Model file for the job. Use its own axes, mm. A direction names the side the tool comes from. Give positions to 0.01 mm unless a question says otherwise; leave off trailing zeros. Loops run counter-clockwise (first coordinate to the right, second up) from the corner with the lowest first, then second, coordinate; pieces in that order, holes last. Notation, with made-up numbers: M 45,9 L 86,9 A27 ccw 86,34 Z; hole C 29,73 d6. An arc over 180 degrees is marked long. Answer in a Markdown table with one row per item.
Autodesk Inventor part; units mm, degrees
ref_plane "Work Plane1" through (-4, 29, 0) normal (0, 1, 0) x (1, 0, 0)
ref_plane "Work Plane2" through (22.5, -4, 10) normal (1, 0, 0) x (0, 0, -1)
ref_plane "YZ Plane" through (0, 0, 0) normal (1, 0, 0) x (0, 1, 0)
sketch "Sketch1" plane through (0, 0, 0) normal (0, 0, 1) x (1, 0, 0)
  line L0 (0, 0) -> (45, 0)
  line L1 (45, 0) -> (45, 58)
  line L2 (45, 58) -> (0, 58)
  line L3 (0, 58) -> (0, 0)
  circle A0 centre (22.5, 53) radius 2.75
  circle A1 centre (22.5, 5) radius 2.75
  line L4 (19.75, 58) -> (19.75, 53)
  line L5 (25.25, 58) -> (25.25, 53)
  line L6 (0, 42) -> (45, 42)
  line L7 (45, 42) -> (45, 16)
  line L8 (45, 16) -> (0, 16)
  line L9 (0, 16) -> (0, 42)
  circle A2 centre (22.5, 53) radius 6
  circle A3 centre (22.5, 5) radius 6
  line L10 (16.5, 5) -> (16.5, -1)
  line L11 (28.5, 5) -> (28.5, -1)
  line L12 (16.5, 53) -> (16.5, 59)
  line L13 (28.5, 53) -> (28.5, 59)
  line L14 (-1, 59) -> (46, 59)
  line L15 (46, 59) -> (46, -1)
  line L16 (46, -1) -> (-1, -1)
  line L17 (-1, -1) -> (-1, 59)
  line L18 (49, 62) -> (-4, 62)
  line L19 (-4, 62) -> (-4, -4)
  line L20 (-4, -4) -> (49, -4)
  line L21 (49, -4) -> (49, 62)
  line L22 (28.5, 59) -> (16.5, 59)
  line L23 (28.5, -1) -> (16.5, -1)
  point P0 (22.5, 58)
  dimension "d0" = 45
  dimension "d1" = 58
  dimension "d2" = 5.5
  dimension "d3" = 5.5
  dimension "d4" = 5
  dimension "d5" = 5
  dimension "d6" = 26
  dimension "d7" = 16
  dimension "d8" = 12
  dimension "d9" = 12
  dimension "d10" = 1
  dimension "d11" = 3
extrude "Extrusion1" add sketch "Sketch1" along normal blind 10 contours L21 L20 L19 L18
sketch "Sketch2" plane through (0, 0, 10) normal (0, 0, 1) x (1, 0, 0)
  line L0 (-1, 59) -> (46, 59)
  line L1 (46, 59) -> (46, -1)
  line L2 (-1, 59) -> (46, 59)
  line L3 (46, 59) -> (46, 43)
  line L4 (46, 43) -> (-1, 43)
  line L5 (-1, 43) -> (-1, 59)
  line L6 (-1, -1) -> (-1, 59)
  line L7 (46, -1) -> (-1, -1)
  line L8 (-1, -1) -> (-1, 15)
  line L9 (-1, 15) -> (46, 15)
  line L10 (46, 15) -> (46, -1)
  point P0 (0, 0)
  dimension "d14" = 16
  dimension "d15" = 16
extrude "Extrusion2" add sketch "Sketch2" against normal blind 3 contours L0 L1 L4 L5 | L9 L1 L7 L6
sketch "Sketch3" plane through (0, 0, 0) normal (0, 0, -1) x (-1, 0, 0)
  arc A0 (-28.5, 53) -> (-16.5, 53) centre (-22.5, 53) ccw
  line L0 (-46, 59) -> (1, 59)
  line L1 (-28.5, 59) -> (-28.5, 53)
  line L2 (-16.5, 59) -> (-16.5, 53)
  line L3 (-16.5, 59) -> (-28.5, 59)
  point P0 (0, 0)
  dimension "d18" = 12
extrude "Extrusion3" add sketch "Sketch3" against normal up to surface (7 mm away)
ref_plane "Work Plane1" through (-4, 29, 0) normal (0, 1, 0) x (1, 0, 0)
mirror "Mirror1" about plane through (-4, 29, 0) normal (0, 1, 0) of "Extrusion3"
thicken "Thicken1" operation add thickness 13 both sides no extend neighbours yes toward (0, 0, -1) faces at (48, 39, 0)
sketch "Sketch4" plane through (-4, 62, 10) normal (0, 1, 0) x (1, 0, 0)
  line L0 (3, 3) -> (3, 0)
  line L1 (3, 0) -> (3, 3)
  line L2 (3, 23) -> (3, 3)
  line L3 (3, 23) -> (3, 3)
  line L4 (50, 0) -> (50, 3)
  line L5 (50, 23) -> (50, 3)
  line L6 (50, 23) -> (50, 3)
  line L7 (50, 3) -> (50, 0)
  line L8 (20.5, 3) -> (32.5, 3)
  line L9 (50, 3) -> (32.5, 3)
  line L10 (50, 3) -> (3, 3)
  line L11 (20.5, 3) -> (3, 3)
  line L12 (32.5, 23) -> (32.5, 3)
  line L13 (32.5, 23) -> (32.5, 3)
  line L14 (20.5, 23) -> (20.5, 3)
  line L15 (20.5, 3) -> (20.5, 23)
  line L16 (53, 23) -> (0, 23)
  line L17 (42, 23) -> (42, 7) construction
  line L18 (38, 23) -> (38, 7)
  line L19 (46, 7) -> (46, 23)
  arc A0 (46, 23) -> (38, 23) centre (42, 23) ccw
  arc A1 (38, 7) -> (46, 7) centre (42, 7) ccw
  point P0 (4, 10)
  point P1 (42, 15)
  dimension "d23" = 4
  dimension "d24" = 8
  dimension "d25" = 16
extrude "Extrusion4" cut sketch "Sketch4" against normal through all contours L16 L19 A1 L18
ref_plane "Work Plane2" through (22.5, -4, 10) normal (1, 0, 0) x (0, 0, -1)
mirror "Mirror2" about plane through (22.5, -4, 10) normal (1, 0, 0) of "Extrusion4"
hole "Hole1" at (22.5, 53, 10) direction (0, 0, -1) diameter 4.5 end through all counterbore diameter 8 counterbore depth 4
mirror "Mirror3" about plane through (-4, 29, 0) normal (0, 1, 0) of "Hole1"
properties part number "ssr-cover"
(1) Saw through at B-B, the plane x = 22.5. Give the cut face in (y, z), and give its area (3 significant figures).
Established:
| item | result |
|---|---|
| outline | M -4,-13 L 2.75,-13 L 2.75,6 L 1,6 L 1,10 L -4,10 Z; M 7.25,-13 L 11,-13 L 11,7 L 15,7 L 15,10 L 9,10 L 9,6 L 7.25,6 Z; M 43,7 L 47,7 L 47,-13 L 50.75,-13 L 50.75,6 L 49,6 L 49,10 L 43,10 Z; M 55.25,-13 L 62,-13 L 62,10 L 57,10 L 57,6 L 55.25,6 Z |
| area | 479 mm2 |
(2) Saw through at D-D, the plane x = 43. Give the cut face in (y, z), and give its area (3 significant figures).
Established:
| item | result |
|---|---|
| outline | M -4,-13 L -1,-13 L -1,7 L 15,7 L 15,10 L -4,10 Z; M 43,7 L 59,7 L 59,-13 L 62,-13 L 62,10 L 43,10 Z |
| area | 234 mm2 |
(3) Mould opens along Y. For faces 5 (the flat face through (23, 62, -2)), 6 (the flat face through (3, -2, -5)), 7 (the flat face through (22, 46, 7)) say: pulls with the +Y half, pulls with the -Y half, needs draft (parallel to the pull), parting line crosses it, or undercut.
Established:
| item | result |
|---|---|
| face 5 | pulls with the +Y half |
| face 6 | needs draft |
| face 7 | undercut |
(4) Saw through at A-A, the plane z = -5.5. Count the separate pieces of the cut face and the enclosed holes in it, and give its area (3 significant figures).
Established:
| item | result |
|---|---|
| separate pieces | 4 |
| enclosed holes | 2 |
| area | 807 mm2 |
(5) Flat gauge pin, fed straight in: P1, Ø1, axis at x = 5, z = -2.5, coming from the -Y side. Where does the tip first touch, or does it go through?
Established:
| item | result |
|---|---|
| P1 | passes through |
(6) Wall check: L1, parallel to Y at x = 22.5, z = -3.5; L2, parallel to Y at x = 22.5, z = 8.6; L3, parallel to X at y = 32.5, z = 7. Give the ranges that are in metal, low to high.
Established:
| item | result |
|---|---|
| L1 | y = -4 to 2.75, 7.25 to 11, 47 to 50.75, 55.25 to 62 |
| L2 | y = -4 to 1, 9 to 15, 43 to 49, 57 to 62 |
| L3 | x = -4 to -1, 46 to 49 |
(7) Saw through at C-C, the plane y = 34. Give the cut face in (x, z).
Established:
| item | result |
|---|---|
| outline | M -4,-13 L -1,-13 L -1,10 L -4,10 Z; M 46,-13 L 49,-13 L 49,10 L 46,10 Z |
(8) Which spindle directions (+Z, -Z, +X, -X, +Y, -Y) get a long thin tool onto all of the face, cutting with end or side? Do faces 1 (the flat face through (42, 61, -5)), 2 (the flat face through (23, 43, 9)), 3 (the flat face through (-1, 29, -2)), 4 (the flat face through (24, 3, 6)). Say none if no direction does.
Established:
| item | result |
|---|---|
| face 1 | -Z, +Y, -Y |
| face 2 | +Z, -Z |
| face 3 | -Z |
| face 4 | +Z |
